from build123d import *

# Parameters (mm, degrees)
F3_D     = 5.2
F3_DEPTH = 8.5
F3_TIP   = 1.5622376095


with BuildPart() as f1:
    # F0 (on Right) → F1 (revolve)
    with BuildSketch(Plane.YZ):
        with BuildLine():
            Line((-36, 5), (-36, 0))
            Line((-36, 0), (0, 0))
            Line((0, 0), (0, 4.7928932188))
            ThreePointArc((0, 4.7928932188), (-0.0380602337, 4.984234935), (-0.1464466094, 5.1464466094))
            Line((-0.1464466094, 5.1464466094), (-1.8535533906, 6.8535533906))
            ThreePointArc((-1.8535533906, 6.8535533906), (-2.015765065, 6.9619397663), (-2.2071067812, 7))
            Line((-2.2071067812, 7), (-28, 7))
            Line((-28, 7), (-28, 5))
            Line((-28, 5), (-36, 5))
        make_face()
    revolve(axis=Axis((0, -18, 0), (0, 1, 0)))

    # F3
    with Locations(Plane.XZ.offset(36)):
        with Locations((0, 0)):
            Hole(F3_D / 2, depth=F3_DEPTH)
            with Locations((0, 0, -(F3_DEPTH + F3_TIP / 2))):  # 118° drill point
                Cone(0, F3_D / 2, F3_TIP, mode=Mode.SUBTRACT)


solid = f1.part
Geometry: final body of the model. Coordinates: model frame, mm. A direction names the side the tool comes from. Round coordinates to 2 decimals unless told otherwise and drop trailing zeros. Order: outer loops, then holes, each group sorted by start corner. A loop starts at its lowest first (then second) coordinate and runs counter-clockwise, first axis right, second up. Notation, with made-up numbers: (77, 74.5) - (82, 74.5) arc R33 ccw to (82, 103.5) - close; hole circle Ø9 at (13.5, 77.25). An arc over 180 degrees is marked (long way). Write each question's results on one line, items separated by ' | '.
Item 1: Reachability of faces 1 (the flat face through (0, 0, 0)), 2 (the cylindrical face through (-4.88, -32.06, -1.08)) from +Z, -Z, +X, -X, +Y, -Y: full face, straight path, thin tool, end or side. Return the list, or none.
Completed:
face 1: +Z, -Z, +X, -X, +Y | face 2: -Y
Item 2: Mould query, pull axis Z, two halves, no side actions, for faces 3 (the flat face through (5, -28, -2)), 4 (the conical face through (-0.36, -26.21, -0.27)), 5 (the conical face through (-5.128, -0.253, -1.139)). Classes: pulls with the +Z half, pulls with the -Z half, needs draft (parallel to the pull), parting line crosses it, or undercut.
Completed:
face 3: needs draft | face 4: undercut | face 5: parting line crosses it
Item 3: Section B-B, the plane y = -20. Return the cut outline in (x, z), and give its area (3 significant figures).
Completed:
outline: circle Ø14 at (0, 0) | area: 154 mm^2
Item 4: Material intervals for line 1 along X through (y, z) = (-33.5, 0); line 2 along Y through (x, z) = (-2.5, 4.5); line 3 along X through (y, z) = (-31, 2.25), sorted ascending. Write a range as [from, to].
Completed:
line 1: [-5, -2.6], [2.6, 5] | line 2: [-28, -0.15] | line 3: [-4.47, -1.3], [1.3, 4.47]
Item 5: Section A-A, the plane y = -32.5. Return the cut outline in (x, z), and give its area (3 significant figures).
Completed:
outline: circle Ø10 at (0, 0); hole circle Ø5.2 at (0, 0) | area: 57.3 mm^2
Item 6: First-contact query: pin 1 Ø3 at (x, y) = (2.5, -20.5) entering from +Z; pin 2 Ø4 at (y, z) = (-23, -5.5) entering from +X; pin 3 Ø4 at (x, y) = (-0.5, -31.5) entering from +Z. Flat tips, straight axial feed; report the tip coordinate or a pass-through.
Completed:
pin 1: z = 6.93 | pin 2: x = 6.06 | pin 3: z = 5
